Geometry check sheet. Reference: drawing and pictorial views, mm from the part's lowest x, y, z. A direction names the side the tool comes from. Give positions to 0.01 mm unless a question says otherwise; leave off trailing zeros. Loops run counter-clockwise (first coordinate to the right, second up) from the corner with the lowest first, then second, coordinate; pieces in that order, holes last. Notation, with made-up numbers: (78.5, 46.25) -> (82.5, 46.25) arc R27 cw to (82.5, 78.25) -> close; hole circle Ø2 at (81, -34). An arc over 180 degrees is marked (long way). One line per item, written item: value. Start each with the question number.
(1) Gauge pin test, flat ends, axial feed: pin 1 Ø4 at (x, y) = (4, 28.5) entering from +Z (1 decimal); pin 2 Ø12 at (y, z) = (18.5, 35) entering from -X; pin 3 Ø6 at (y, z) = (21, 15) entering from -X; pin 4 Ø4 at (x, z) = (3.69, 9.69) entering from -Y. Record the tip position at first contact, or that the pin passes through.
(2) Sectioned sample at B-B, the plane x = 16. Record the cut outline in (y, z) (1 decimal), then the cut area to 3 significant figures.
(3) Tool access check on the marked faces 1 and 2. Record the directions out of +Z, -Z, +X, -X, +Y, -Y that give a thin tool (end or side, any length) a straight path to the whole face; none if there is none.
(4) Sectioned sample at D-D, the plane z = 11. Record the cut outline in (x, y) (1 decimal).
(5) Draft check along X on the marked faces 3, 4 and 5. Enter one of: pulls with the +X half, pulls with the -X half, needs draft (parallel to the pull), parting line crosses it, or undercut.
(6) Scan lines: line 1 along X through (y, z) = (28, 19) (1 decimal); line 2 along X through (y, z) = (26, 23.5); line 3 along Y through (x, z) = (19, 3). Record each from-to range of solid material in increasing order. Write a range as from..to.
(7) Sectioned sample at C-C, the plane y = 5. Record the cut outline in (x, z).
(8) Sectioned sample at A-A, the plane z = 21. Record the cut outline in (x, y).
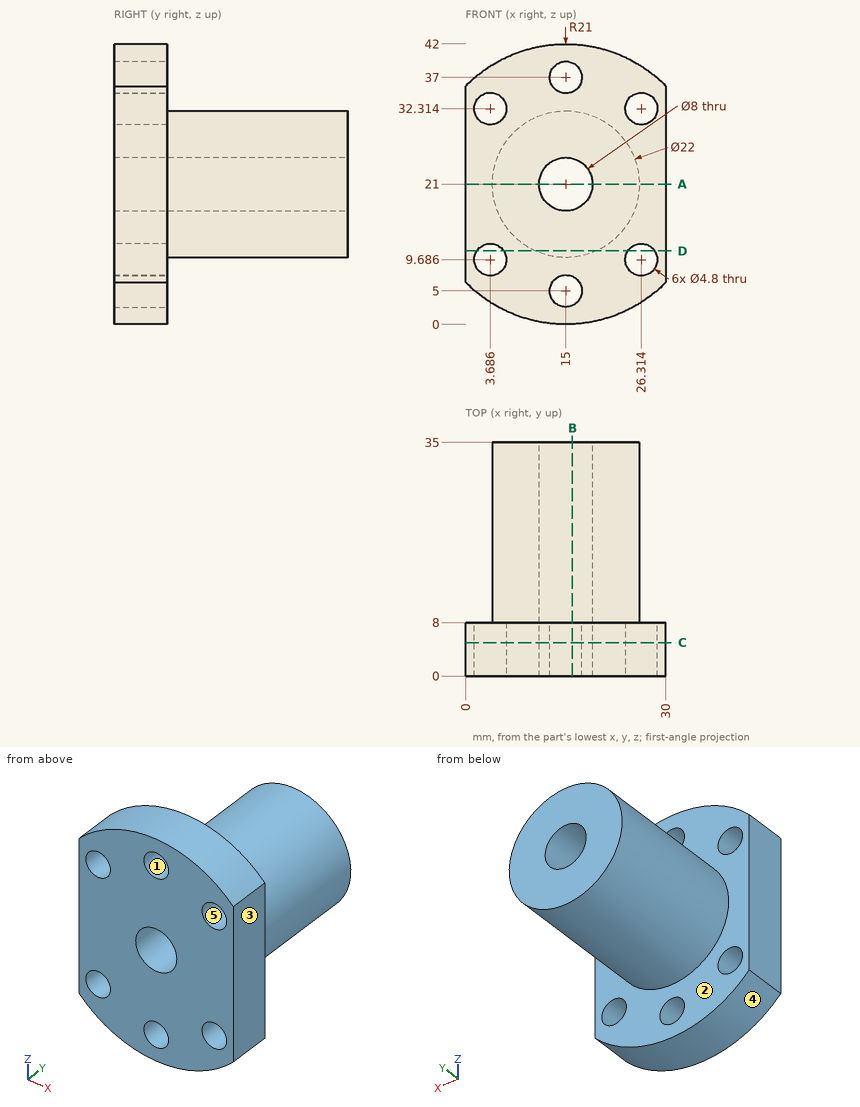
Calculated:
1. pin 1: stops at z = 27.3
1. pin 2: stops at x = 7.45
1. pin 3: stops at x = 4.42
1. pin 4: passes through
2. outline: (0, 0) -> (8, 0) -> (8, 2.8) -> (0, 2.8) -> close; (0, 7.2) -> (8, 7.2) -> (8, 10) -> (35, 10) -> (35, 17.1) -> (0, 17.1) -> close; (0, 24.9) -> (35, 24.9) -> (35, 32) -> (8, 32) -> (8, 34.8) -> (0, 34.8) -> close; (0, 39.2) -> (8, 39.2) -> (8, 42) -> (0, 42) -> close
2. area: 586 mm2
3. face 1: +Y, -Y
3. face 2: +Y
4. outline: (0, 0) -> (1.7, 0) -> (1.7, 8) -> (0, 8) -> close; (5.7, 0) -> (24.3, 0) -> (24.3, 8) -> (19.6, 8) -> (19.6, 35) -> (10.4, 35) -> (10.4, 8) -> (5.7, 8) -> close; (28.3, 0) -> (30, 0) -> (30, 8) -> (28.3, 8) -> close
5. face 3: pulls with the +X half
5. face 4: parting line crosses it
5. face 5: undercut
6. line 1: x = 4.2..11.5, 18.5..25.8
6. line 2: x = 4.29..11.88, 18.12..25.71
6. line 3: y = 0..8
7. outline: (0, 6.3) arc R21 ccw to (30, 6.3) -> (30, 35.7) arc R21 ccw to (0, 35.7) -> close; hole circle Ø4.8 at (3.69, 9.69); hole circle Ø4.8 at (3.69, 32.31); hole circle Ø8 at (15, 21); hole circle Ø4.8 at (15, 5); hole circle Ø4.8 at (15, 37); hole circle Ø4.8 at (26.31, 9.69); hole circle Ø4.8 at (26.31, 32.31)
8. outline: (0, 0) -> (11, 0) -> (11, 35) -> (4, 35) -> (4, 8) -> (0, 8) -> close; (19, 0) -> (30, 0) -> (30, 8) -> (26, 8) -> (26, 35) -> (19, 35) -> close
